Verification items for this drawing (mm, ordinates from the low corner). Give positions to 0.01 mm unless a question says otherwise; leave off trailing zeros. Loops run counter-clockwise (first coordinate to the right, second up) from the corner with the lowest first, then second, coordinate; pieces in that order, holes last. Notation, with made-up numbers: (82, 78) -> (105, 78) arc R27 ccw to (105, 106) -> close; hole circle Ø4 at (-27, 14). An arc over 180 degrees is marked (long way). Answer as CSV lines item,"result". Start each with the question number.
(1) Section check B-B on y = 1.6. Enter the section's corners in (x, z).
(2) Material ranges on line 1 (X direction, y = 1.55, z = 2.2); line 2 (X direction, y = 2.05, z = 1.95) (1 decimal); line 3 (X direction, y = 4.55, z = 4.2), recorded low to high. Write a range as from..to.
(3) Gauge pin test, flat ends, axial feed: pin 1 Ø1.5 at (y, z) = (3.5, 2.5) entering from +X; pin 2 Ø2.5 at (x, z) = (150, 3.5) entering from +Y. Record the tip position at first contact, or that the pin passes through.
(4) Section check A-A on z = 2.45. Enter the section's corners in (x, y), plus the area to 3 significant figures.
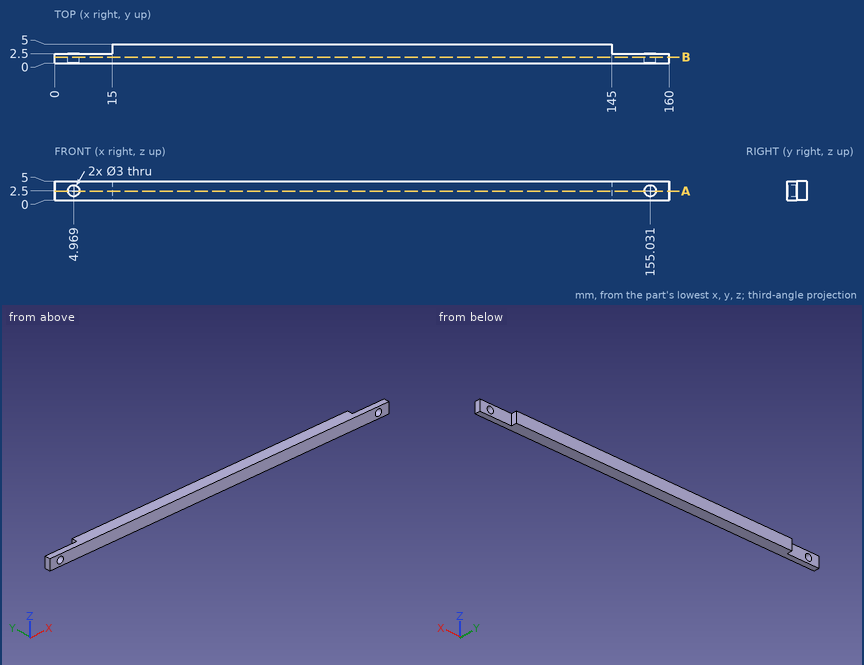
Working result:
1,outline,"(0, 0) -> (160, 0) -> (160, 5) -> (0, 5) -> close; hole circle Ø3 at (4.97, 2.5); hole circle Ø3 at (155.03, 2.5)"
2,line 1,"x = 0..3.5, 6.44..153.56, 156.5..160"
2,line 2,"x = 0..3.6, 6.4..153.6, 156.4..160"
2,line 3,"x = 15..145"
3,pin 1,"stops at x = 145"
3,pin 2,"stops at y = 2.5"
4,outline,"(0, 0) -> (3.47, 0) -> (3.47, 2.5) -> (0, 2.5) -> close; (6.47, 0) -> (153.53, 0) -> (153.53, 2.5) -> (145, 2.5) -> (145, 5) -> (15, 5) -> (15, 2.5) -> (6.47, 2.5) -> close; (156.53, 0) -> (160, 0) -> (160, 2.5) -> (156.53, 2.5) -> close"
4,area,"710 mm^2"
